```python
from build123d import *

# Parameters (mm, degrees)
SKETCH_1_R               = 12
EXTRUDE_1_DEPTH          = 44
CUT_EXTRUDE_1_DEPTH      = 48.15930449
CUT_EXTRUDE_1_DEPTH_BACK = 48.15930449
SKETCH_2_R               = 6
CHAMFER_1_SIZE           = 1
CUT_EXTRUDE_2_DEPTH      = 48.15930449
CUT_EXTRUDE_2_DEPTH_BACK = 48.15930449


with BuildPart() as part:
    # 草图1 → 凸台-拉伸1 (new body)
    with BuildSketch(Plane.XY):
        Circle(SKETCH_1_R)
    extrude(amount=EXTRUDE_1_DEPTH)

    # 草图2 → 切除-拉伸1 (cut, two sides: drawn at the far end of the back side and taken through both)
    with BuildSketch(Plane.XY.offset(44).offset(-CUT_EXTRUDE_1_DEPTH_BACK)):
        Circle(SKETCH_2_R)
    extrude(amount=CUT_EXTRUDE_1_DEPTH + CUT_EXTRUDE_1_DEPTH_BACK, mode=Mode.SUBTRACT)

    # 倒角1
    chamfer_1_edges = [part.edges().sort_by_distance(p)[0] for p in [
        (-12, 0, 0),
        (-12, 0, 44),
    ]]
    chamfer(chamfer_1_edges, length=CHAMFER_1_SIZE)

    # 草图3 → 切除-拉伸2 (cut, two sides: drawn at the far end of the back side and taken through both)
    with BuildSketch(Plane(origin=(0, 0, 0), x_dir=(0, 0, -1), z_dir=(1, 0, 0)).offset(-CUT_EXTRUDE_2_DEPTH_BACK)):
        with BuildLine():
            Line((-62.986172875, 133.10063067), (-25.120459682, 29.369909319))
            ThreePointArc((-25.120459682, 29.369909319), (-14.752953683, 15.315455683), (1.566572924, 9.095656735))
            Line((1.566572924, 9.095656735), (111.651710823, 0.427484986))
            Line((111.651710823, 0.427484986), (245.252446132, 176.286356459))
            Line((245.252446132, 176.286356459), (70.614562433, 308.959502143))
            Line((70.614562433, 308.959502143), (-62.986172875, 133.10063067))
        make_face()
    extrude(amount=CUT_EXTRUDE_2_DEPTH + CUT_EXTRUDE_2_DEPTH_BACK, mode=Mode.SUBTRACT)


solid = part.part
```
Could you check a few things on this model? Use its own coordinates, in mm. Round coordinates to 2 decimals unless told otherwise and drop trailing zeros. Loops run counter-clockwise (first coordinate to the right, second up) from the corner with the lowest first, then second, coordinate; pieces in that order, holes last. Notation, with made-up numbers: (77, 46.25) - (109, 46.25) arc R25 ccw to (109, 62.25) - close; hole circle Ø6 at (-24, 59.5). An arc over 180 degrees is marked (long way). Answer in a Markdown table with one row per item. Add a question column.
(1) If we section it at A-A (x = 0): Please give me the cut outline in (y, z), plus the area to 3 significant figures.
(2) If we section it at B-B (y = 0): Please give me the cut outline in (x, z).
(3) If we section it at C-C (z = 41.5): Please give me the cut outline in (x, y), plus the area to 3 significant figures.
(4) I need wall thicknesses on line 1 along X through (y, z) = (0, 25); line 2 along Y through (x, z) = (-5.25, 18.5). Which ranges of each line are inside material? Lowest first, please.
(5) If we mould it in two halves opening along Y, with no side actions, what happens to faces 1 (the face through (-6, 0, 22)), 2 (the face through (-0.104, 9.993, 3.783)), 3 (the face through (5, -5, 44))? For each: pulls with the +Y half, pulls with the -Y half, needs draft (parallel to the pull), parting line crosses it, or undercut.
(6) I'm going to push flat-ended pins straight in: pin 1 (2 mm diameter, centred on x = -3, y = 3, fed in from +Z); pin 2 (12 mm diameter, centred on x = 4, z = 19, fed in from +Y); pin 3 (12 mm diameter, centred on x = 6.5, z = 37.5, fed in from -Y); pin 4 (1.5 mm diameter, centred on x = 4, z = 19.5, fed in from +Y). Where does each tip first touch, or does it pass through?
Model answer:
| question | item | result |
|---|---|---|
| 1 | outline | (-12, 1) - (-11, 0) - (-6, 0) - (-6, 44) - (-11, 44) - (-12, 43) - close; (6, 0) - (9.26, 0) arc R31 cw to (12, 9.3) - (12, 43) - (11, 44) - (6, 44) - close |
| 1 | area | 511 mm² |
| 2 | outline | (-12, 1) - (-11, 0) - (-6, 0) - (-6, 44) - (-11, 44) - (-12, 43) - close; (6, 0) - (11, 0) - (12, 1) - (12, 43) - (11, 44) - (6, 44) - close |
| 3 | outline | circle Ø24 at (0, 0); hole circle Ø12 at (0, 0) |
| 3 | area | 339 mm² |
| 4 | line 1 | x = -12 to -6, 6 to 12 |
| 4 | line 2 | y = -10.79 to -2.9, 2.9 to 10.79 |
| 5 | face 1 | undercut |
| 5 | face 2 | pulls with the +Y half |
| 5 | face 3 | needs draft |
| 6 | pin 1 | passes through |
| 6 | pin 2 | stops at y = 12 |
| 6 | pin 3 | stops at y = -11.99 |
| 6 | pin 4 | stops at y = 11.55 |
